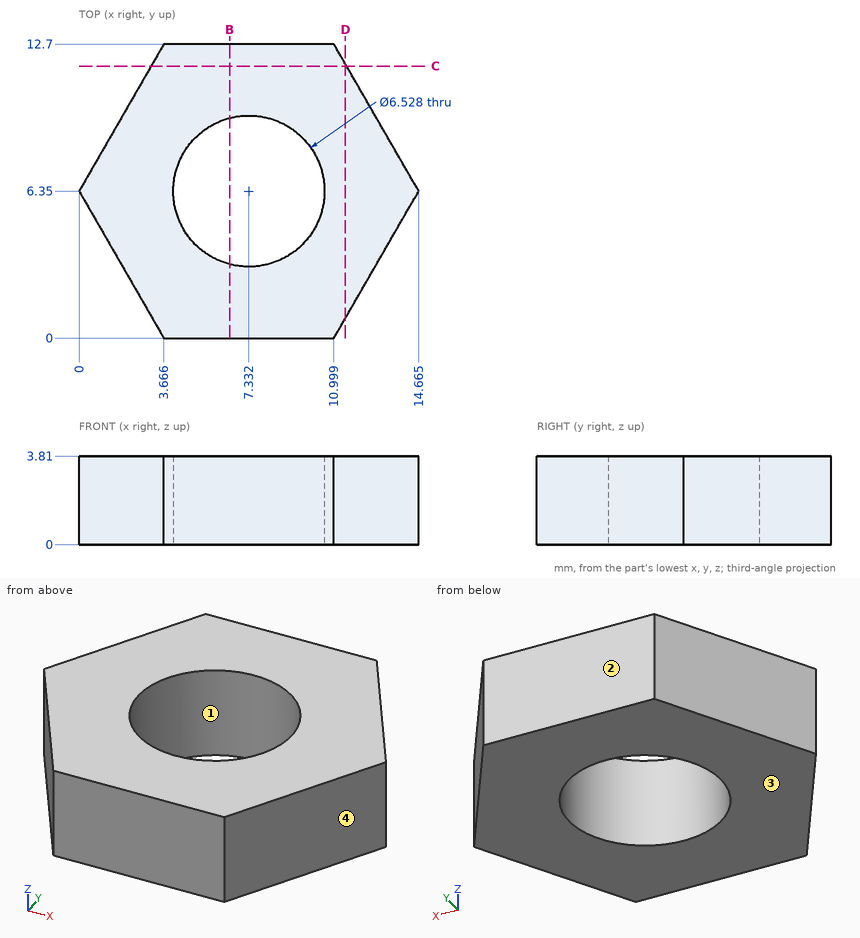
Input: dimensioned drawing with shaded views. Units: mm. Origin: part minimum x, y, z. Give positions to 0.01 mm unless a question says otherwise; leave off trailing zeros. Order: outer loops, then holes, each group sorted by start corner. A loop starts at its lowest first (then second) coordinate and runs counter-clockwise, first axis right, second up. Notation, with made-up numbers: (25, 16.5) -> (76, 16.5) arc R15 cw to (76, 28.5) -> close; hole circle Ø8 at (-35.5, 13.25). An arc over 180 degrees is marked (long way). Use one line per item in the form item = value.
1) Section D-D, the plane x = 11.5. Return loops of the section in (y, z).
Response values:
outline = (0.87, 0) -> (11.83, 0) -> (11.83, 3.81) -> (0.87, 3.81) -> close
2) Section C-C, the plane y = 11.75. Return loops of the section in (x, z), and give its area (3 significant figures).
Response values:
outline = (3.12, 0) -> (11.55, 0) -> (11.55, 3.81) -> (3.12, 3.81) -> close
area = 32.1 mm^2
3) Section B-B, the plane x = 6.5. Return loops of the section in (y, z).
Response values:
outline = (0, 0) -> (3.19, 0) -> (3.19, 3.81) -> (0, 3.81) -> close; (9.51, 0) -> (12.7, 0) -> (12.7, 3.81) -> (9.51, 3.81) -> close
4) Mould query, pull axis Y, two halves, no side actions, for the marked faces 1, 2, 3 and 4. Classes: pulls with the +Y half, pulls with the -Y half, needs draft (parallel to the pull), parting line crosses it, or undercut.
Response values:
face_1 = undercut
face_2 = pulls with the +Y half
face_3 = needs draft
face_4 = pulls with the -Y half
5) First-contact query: pin 1 Ø1.5 at (y, z) = (1.5, 2) entering from +X. Flat tip, straight axial feed; report the tip coordinate or a pass-through.
Response values:
pin_1 = 12.3
6) Line query: probe 1 along X at (y, z) = (6.25, 3.25) (1 decimal); probe 2 along X at (y, z) = (5, 3.3) (1 decimal); probe 3 along Y at (x, z) = (9.75, 0.45) (1 decimal). Output: solid intervals per line, ascending.
Response values:
probe_1 = 0.1 to 4.1, 10.6 to 14.6
probe_2 = 0.8 to 4.4, 10.3 to 13.9
probe_3 = 0 to 4.2, 8.5 to 12.7
